```python
from build123d import *

# Parameters (mm, degrees)
SKETCH1_R           = 6
SKETCH1_W           = 10
SKETCH1_H           = 3.175
SKETCH1_W_2         = 192
SKETCH1_H_2         = 96
BOSS_EXTRUDE1_DEPTH = 3.175


with BuildPart() as part:
    # Sketch1 → Boss-Extrude1 (new body)
    with BuildSketch(Plane(origin=(0, 0, 0), x_dir=(1, 0, 0), z_dir=(0, 1, 0))):
        Polygon((0, 145), (0, 160), (252, 160), (252, 145), (255.175, 145), (255.175, 135), (252, 135), (252, 125), (255.175, 125), (255.175, 115), (252, 115), (252, 105), (255.175, 105), (255.175, 95), (252, 95), (252, 85), (255.175, 85), (255.175, 75), (252, 75), (252, 65), (255.175, 65), (255.175, 55), (252, 55), (252, 45), (255.175, 45), (255.175, 35), (252, 35), (252, 25), (255.175, 25), (255.175, 15), (252, 15), (252, 0), (0, 0), (0, 15), (-3.175, 15), (-3.175, 25), (0, 25), (0, 35), (-3.175, 35), (-3.175, 45), (0, 45), (0, 55), (-3.175, 55), (-3.175, 65), (0, 65), (0, 75), (-3.175, 75), (-3.175, 85), (0, 85), (0, 95), (-3.175, 95), (-3.175, 105), (0, 105), (0, 115), (-3.175, 115), (-3.175, 125), (0, 125), (0, 135), (-3.175, 135), (-3.175, 145), align=None)
        with Locations((106, 24)):
            Circle(SKETCH1_R, mode=Mode.SUBTRACT)
        with Locations((66, 24)):
            Circle(SKETCH1_R, mode=Mode.SUBTRACT)
        with Locations((186, 24)):
            Circle(SKETCH1_R, mode=Mode.SUBTRACT)
        with Locations((146, 24)):
            Circle(SKETCH1_R, mode=Mode.SUBTRACT)
        with Locations((36, 155.4125)):
            Rectangle(SKETCH1_W, SKETCH1_H, mode=Mode.SUBTRACT)
        with Locations((126, 87)):
            Rectangle(SKETCH1_W_2, SKETCH1_H_2, mode=Mode.SUBTRACT)
        with Locations((16, 155.4125)):
            Rectangle(SKETCH1_W, SKETCH1_H, mode=Mode.SUBTRACT)
        with Locations((56, 155.4125)):
            Rectangle(SKETCH1_W, SKETCH1_H, mode=Mode.SUBTRACT)
        with Locations((76, 155.4125)):
            Rectangle(SKETCH1_W, SKETCH1_H, mode=Mode.SUBTRACT)
        with Locations((96, 155.4125)):
            Rectangle(SKETCH1_W, SKETCH1_H, mode=Mode.SUBTRACT)
        with Locations((116, 155.4125)):
            Rectangle(SKETCH1_W, SKETCH1_H, mode=Mode.SUBTRACT)
        with Locations((136, 155.4125)):
            Rectangle(SKETCH1_W, SKETCH1_H, mode=Mode.SUBTRACT)
        with Locations((156, 155.4125)):
            Rectangle(SKETCH1_W, SKETCH1_H, mode=Mode.SUBTRACT)
        with Locations((176, 155.4125)):
            Rectangle(SKETCH1_W, SKETCH1_H, mode=Mode.SUBTRACT)
        with Locations((196, 155.4125)):
            Rectangle(SKETCH1_W, SKETCH1_H, mode=Mode.SUBTRACT)
        with Locations((216, 155.4125)):
            Rectangle(SKETCH1_W, SKETCH1_H, mode=Mode.SUBTRACT)
        with Locations((236, 155.4125)):
            Rectangle(SKETCH1_W, SKETCH1_H, mode=Mode.SUBTRACT)
        with Locations((236, 4.5875)):
            Rectangle(SKETCH1_W, SKETCH1_H, mode=Mode.SUBTRACT)
        with Locations((216, 4.5875)):
            Rectangle(SKETCH1_W, SKETCH1_H, mode=Mode.SUBTRACT)
        with Locations((196, 4.5875)):
            Rectangle(SKETCH1_W, SKETCH1_H, mode=Mode.SUBTRACT)
        with Locations((176, 4.5875)):
            Rectangle(SKETCH1_W, SKETCH1_H, mode=Mode.SUBTRACT)
        with Locations((156, 4.5875)):
            Rectangle(SKETCH1_W, SKETCH1_H, mode=Mode.SUBTRACT)
        with Locations((136, 4.5875)):
            Rectangle(SKETCH1_W, SKETCH1_H, mode=Mode.SUBTRACT)
        with Locations((116, 4.5875)):
            Rectangle(SKETCH1_W, SKETCH1_H, mode=Mode.SUBTRACT)
        with Locations((96, 4.5875)):
            Rectangle(SKETCH1_W, SKETCH1_H, mode=Mode.SUBTRACT)
        with Locations((76, 4.5875)):
            Rectangle(SKETCH1_W, SKETCH1_H, mode=Mode.SUBTRACT)
        with Locations((56, 4.5875)):
            Rectangle(SKETCH1_W, SKETCH1_H, mode=Mode.SUBTRACT)
        with Locations((36, 4.5875)):
            Rectangle(SKETCH1_W, SKETCH1_H, mode=Mode.SUBTRACT)
        with Locations((16, 4.5875)):
            Rectangle(SKETCH1_W, SKETCH1_H, mode=Mode.SUBTRACT)
    extrude(amount=BOSS_EXTRUDE1_DEPTH)


solid = part.part
```
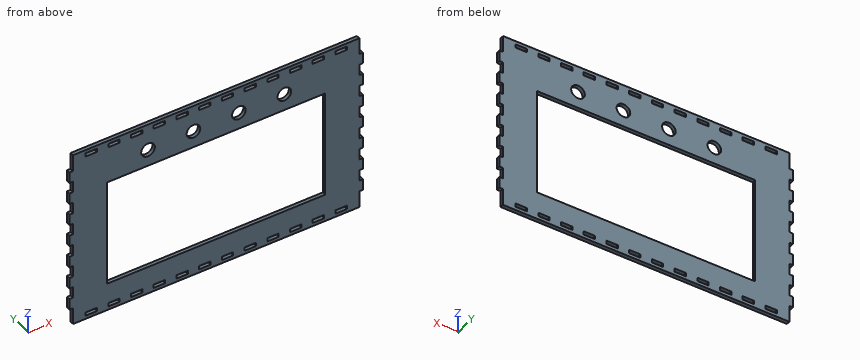
For this review, take the finished solid that the model builds, in its own axes (mm). Coordinates: 2 decimals unless noted, no trailing zeros. Loops run counter-clockwise (first coordinate to the right, second up) from the corner with the lowest first, then second, coordinate; pieces in that order, holes last. Notation, with made-up numbers: (-5.75, 58) -> (23.25, 58) arc R13 ccw to (23.25, 65) -> close; hole circle Ø10 at (48, -11). An arc over 180 degrees is marked (long way). Return JSON: item names as keys, results as strings. Group by question number.
(1) Consider section D-D, the plane y = 2.65. Count the separate pieces of the cut face and the enclosed holes in it, plus the area to 3 significant figures.
(2) Consider section A-A, the plane x = 165. Give the boundary of the cut face in (y, z) (3 decimals), plus the area to 3 significant figures.
(3) To check wall thickness, follow L1, parallel to Z at x = 106, y = 1.1; L2, parallel to Z at x = 94, y = 1 (3 decimals); L3, parallel to X at y = 1.4, z = -24 (3 decimals). State the ranges of each line that lie inside material, in increasing order.
(4) For pin 1 Ø1 at (y, z) = (2, -155.5) entering from -X; pin 2 Ø1 at (y, z) = (2, -5) entering from +X; pin 3 Ø1 at (x, y) = (-1.5, 1.5) entering from -Z, all flat-tipped, find the tip position at first contact; note any pin that passes through.
(5) Consider section C-C, the plane x = 63.5. Give the boundary of the cut face in (y, z) (3 decimals).
(6) Consider section B-B, the plane z = -78. Give the boundary of the cut face in (x, y) (3 decimals).
Results below:
{
 "1": {"separate pieces": "1", "enclosed holes": "29", "area": "21,100 mm2"},
 "2": {"outline": "(0, -160) -> (3.175, -160) -> (3.175, -135) -> (0, -135) -> close; (0, -39) -> (3.175, -39) -> (3.175, 0) -> (0, 0) -> close", "area": "203 mm2"},
 "3": {"L1": "z = -160 to -135, -39 to -30, -18 to 0", "L2": "z = -160 to -157, -153.825 to -135, -39 to -6.175, -3 to 0", "L3": "x = -3.175 to 60, 72 to 100, 112 to 140, 152 to 180, 192 to 255.175"},
 "4": {"pin 1": "stops at x = 0", "pin 2": "stops at x = 252", "pin 3": "stops at z = -145"},
 "5": {"outline": "(0, -160) -> (3.175, -160) -> (3.175, -135) -> (0, -135) -> close; (0, -39) -> (3.175, -39) -> (3.175, -29.454) -> (0, -29.454) -> close; (0, -18.546) -> (3.175, -18.546) -> (3.175, 0) -> (0, 0) -> close"},
 "6": {"outline": "(-3.175, 0) -> (30, 0) -> (30, 3.175) -> (-3.175, 3.175) -> close; (222, 0) -> (255.175, 0) -> (255.175, 3.175) -> (222, 3.175) -> close"}
}
